Check sheet for the modelled part. Datum: model origin and axes. Units: mm. A direction names the side the tool comes from. Coordinates: 2 decimals unless noted, no trailing zeros. Write each loop counter-clockwise with the first axis right and the second up, starting at its lowest first coordinate (ties: lowest second). Pieces come first, ordered by that corner, then holes. Notation, with made-up numbers: M 24,48 L 65,48 A29 ccw 65,81 Z; hole C -11.5,12.5 d8. An arc over 180 degrees is marked long. Answer as CSV lines item,"result". Start each with the question number.
Q1. Mould release check, pull along X, two halves, no side actions. Record for faces 3 (the flat face through (74, 0, 5)), 4 (the flat face through (150, 111, 5)), 5 (the cylindrical face through (10.17, 135.48, 5.07)): pulls with the +X half, pulls with the -X half, needs draft (parallel to the pull), parting line crosses it, or undercut.
Q2. Sectioned sample at C-C, the plane x = 98. Record the cut outline in (y, z).
Q3. Sectioned sample at A-A, the plane y = 61. Record the cut outline in (x, z).
Q4. Thickness scan on line 1 along Y through (x, z) = (98, 3.5); line 2 along X through (y, z) = (133, 7); line 3 along Y through (x, z) = (53, 1). Record the ranges inside material, lowest first. Write a range as from..to.
Q5. Sectioned sample at D-D, the plane y = 116. Record the cut outline in (x, z), then the cut area to 3 significant figures.
Q6. Depth check by flat-ended pin: pin 1 Ø3 at (x, y) = (10.5, 133) entering from -Z; pin 2 Ø2.5 at (x, y) = (65.5, 115) entering from +Z. Enter the tip coordinate at first touch or a pass-through.
Q7. Sectioned sample at B-B, the plane x = 64. Record the cut outline in (y, z).
Q8. Access from +Z, -Z, +X, -X, +Y, -Y to the whole of each face (thin tool, end or side, straight path). Record for faces 1 (the cylindrical face through (85.479, 119.966, 7.535)), 2 (the cylindrical face through (98, 220, 5)).
from build123d import *

# Parameters (mm, degrees)
CROQUIS1_W              = 150
CROQUIS1_H              = 225
SALIENTE_EXTRUIR1_DEPTH = 10
CROQUIS2_R              = 2.5
CORTAR_EXTRUIR1_DEPTH   = 271.601182555
CROQUIS3_R              = 3
CORTAR_EXTRUIR3_DEPTH   = 271.601182555
CROQUIS6_R              = 4
CORTAR_EXTRUIR5_DEPTH   = 5
CROQUIS7_R              = 2
CORTAR_EXTRUIR6_DEPTH   = 271.601182555
CROQUIS8_R              = 3
CORTAR_EXTRUIR7_DEPTH   = 271.601182555


with BuildPart() as part:
    # Croquis1 → Saliente-Extruir1 (new body)
    with BuildSketch(Plane.XY):
        with Locations((75, 112.5)):
            Rectangle(CROQUIS1_W, CROQUIS1_H)
    extrude(amount=SALIENTE_EXTRUIR1_DEPTH)

    # Croquis2 → Cortar-Extruir1 (cut, through all)
    with BuildSketch(Plane.XY.offset(10)):
        with Locations((10.5, 169)):
            Circle(CROQUIS2_R)
        with Locations((40.5, 169)):
            Circle(CROQUIS2_R)
        with Locations((10.5, 133)):
            Circle(CROQUIS2_R)
        with Locations((40.5, 133)):
            Circle(CROQUIS2_R)
        with Locations(Location((109.5, 133, 0), (0, 0, 180))):
            Circle(CROQUIS2_R)
        with Locations(Location((109.5, 169, 0), (0, 0, 180))):
            Circle(CROQUIS2_R)
        with Locations(Location((139.5, 133, 0), (0, 0, 180))):
            Circle(CROQUIS2_R)
        with Locations(Location((139.5, 169, 0), (0, 0, 180))):
            Circle(CROQUIS2_R)
        with Locations((139.5, 61)):
            Circle(CROQUIS2_R)
        with Locations((109.5, 61)):
            Circle(CROQUIS2_R)
        with Locations((139.5, 25)):
            Circle(CROQUIS2_R)
        with Locations((109.5, 25)):
            Circle(CROQUIS2_R)
        with Locations(Location((40.5, 61, 0), (0, 0, 180))):
            Circle(CROQUIS2_R)
        with Locations(Location((40.5, 25, 0), (0, 0, 180))):
            Circle(CROQUIS2_R)
        with Locations(Location((10.5, 61, 0), (0, 0, 180))):
            Circle(CROQUIS2_R)
        with Locations(Location((10.5, 25, 0), (0, 0, 180))):
            Circle(CROQUIS2_R)
    extrude(amount=-CORTAR_EXTRUIR1_DEPTH, mode=Mode.SUBTRACT)

    # Croquis3 → Cortar-Extruir3 (cut, through all)
    with BuildSketch(Plane.XY.offset(10)):
        with Locations((64, 116)):
            Circle(CROQUIS3_R)
        with Locations((64, 78)):
            Circle(CROQUIS3_R)
        with Locations((86, 78)):
            Circle(CROQUIS3_R)
        with Locations((86, 116)):
            Circle(CROQUIS3_R)
    extrude(amount=-CORTAR_EXTRUIR3_DEPTH, mode=Mode.SUBTRACT)

    # Croquis6 → Cortar-Extruir5 (cut)
    with BuildSketch(Plane.XY.offset(10)):
        with Locations((64, 116)):
            Circle(CROQUIS6_R)
        with Locations((64, 78)):
            Circle(CROQUIS6_R)
        with Locations((86, 78)):
            Circle(CROQUIS6_R)
        with Locations((86, 116)):
            Circle(CROQUIS6_R)
    extrude(amount=-CORTAR_EXTRUIR5_DEPTH, mode=Mode.SUBTRACT)

    # Croquis7 → Cortar-Extruir6 (cut, through all)
    with BuildSketch(Plane(origin=(0, 0, 0), x_dir=(-1, 0, 0), z_dir=(0, 0, -1))):
        with Locations((-143, 216)):
            Circle(CROQUIS7_R)
        with Locations((-111, 216)):
            Circle(CROQUIS7_R)
        with Locations(Location((-39, 216, 0), (0, 0, 180))):
            Circle(CROQUIS7_R)
        with Locations(Location((-7, 216, 0), (0, 0, 180))):
            Circle(CROQUIS7_R)
        with Locations((-7, 9)):
            Circle(CROQUIS7_R)
        with Locations((-39, 9)):
            Circle(CROQUIS7_R)
        with Locations(Location((-111, 9, 0), (0, 0, 180))):
            Circle(CROQUIS7_R)
        with Locations(Location((-143, 9, 0), (0, 0, 180))):
            Circle(CROQUIS7_R)
    extrude(amount=-CORTAR_EXTRUIR6_DEPTH, mode=Mode.SUBTRACT)

    # Croquis8 → Cortar-Extruir7 (cut, through all)
    with BuildSketch(Plane(origin=(0, 0, 0), x_dir=(-1, 0, 0), z_dir=(0, 0, -1))):
        with Locations((-98, 217)):
            Circle(CROQUIS8_R)
        with Locations((-52, 217)):
            Circle(CROQUIS8_R)
        with Locations((-98, 204)):
            Circle(CROQUIS8_R)
        with Locations((-52, 204)):
            Circle(CROQUIS8_R)
        with Locations((-98, 53)):
            Circle(CROQUIS8_R)
        with Locations((-52, 53)):
            Circle(CROQUIS8_R)
    extrude(amount=-CORTAR_EXTRUIR7_DEPTH, mode=Mode.SUBTRACT)


solid = part.part
Output:
1,face 3,"needs draft"
1,face 4,"pulls with the +X half"
1,face 5,"undercut"
2,outline,"M 0,0 L 50,0 L 50,10 L 0,10 Z; M 56,0 L 201,0 L 201,10 L 56,10 Z; M 207,0 L 214,0 L 214,10 L 207,10 Z; M 220,0 L 225,0 L 225,10 L 220,10 Z"
3,outline,"M 0,0 L 8,0 L 8,10 L 0,10 Z; M 13,0 L 38,0 L 38,10 L 13,10 Z; M 43,0 L 107,0 L 107,10 L 43,10 Z; M 112,0 L 137,0 L 137,10 L 112,10 Z; M 142,0 L 150,0 L 150,10 L 142,10 Z"
4,line 1,"y = 0..50, 56..201, 207..214, 220..225"
4,line 2,"x = 0..8, 13..38, 43..107, 112..137, 142..150"
4,line 3,"y = 0..50.17, 55.83..201.17, 206.83..214.17, 219.83..225"
5,outline,"M 0,0 L 61,0 L 61,5 L 60,5 L 60,10 L 0,10 Z; M 67,0 L 83,0 L 83,5 L 82,5 L 82,10 L 68,10 L 68,5 L 67,5 Z; M 89,0 L 150,0 L 150,10 L 90,10 L 90,5 L 89,5 Z"
5,area,"1,360 mm^2"
6,pin 1,"passes through"
6,pin 2,"stops at z = 5"
7,outline,"M 0,0 L 75,0 L 75,5 L 74,5 L 74,10 L 0,10 Z; M 81,0 L 113,0 L 113,5 L 112,5 L 112,10 L 82,10 L 82,5 L 81,5 Z; M 119,0 L 225,0 L 225,10 L 120,10 L 120,5 L 119,5 Z"
8,face 1,"+Z"
8,face 2,"+Z, -Z"
